```python
from build123d import *

# Parameters (mm, degrees)
F0_R     = 1.6
F1_DEPTH = 3.175


with BuildPart() as f1:
    # F0 (on Top) → F1 (new body)
    with BuildSketch(Plane.XY):
        with BuildLine():
            ThreePointArc((0, 10), (2.928932, 2.928932), (10, 0))
            Line((10, 0), (46, 0))
            ThreePointArc((46, 0), (49.535534, 1.464466), (51, 5))
            Line((51, 5), (51, 15))
            ThreePointArc((51, 15), (49.535534, 18.535534), (46, 20))
            Line((46, 20), (10, 20))
            ThreePointArc((10, 20), (2.928932, 17.071068), (0, 10))
        make_face()
        with Locations((16, 5)):
            Circle(F0_R, mode=Mode.SUBTRACT)
        with Locations((26, 5)):
            Circle(F0_R, mode=Mode.SUBTRACT)
        with Locations((36, 5)):
            Circle(F0_R, mode=Mode.SUBTRACT)
        with Locations((46, 5)):
            Circle(F0_R, mode=Mode.SUBTRACT)
        Polygon((5.686873, 11.150841), (5.518811, 11.651718), (6.045746, 11.689937), (6.007527, 12.216873), (6.527413, 12.122848), (6.621438, 12.642733), (7.101608, 12.422372), (7.321969, 12.902541), (7.732252, 12.56969), (8.065104, 12.979972), (8.37972, 12.555544), (8.804147, 12.87016), (9.003328, 12.380825), (9.492663, 12.580005), (9.563894, 12.056509), (10.08739, 12.12774), (10.026194, 11.602976), (10.550958, 11.54178), (10.361181, 11.048721), (10.85424, 10.858945), (10.547807, 10.428572), (10.97818, 10.122139), (10.574344, 9.781494), (10.914989, 9.377658), (10.439126, 9.148145), (10.668639, 8.672282), (10.150649, 8.568322), (10.254609, 8.050331), (9.727038, 8.078456), (9.698914, 7.550885), (9.194912, 7.709328), (9.036469, 7.205326), (8.587704, 7.484131), (8.308899, 7.035366), (7.943569, 7.417015), (7.56192, 7.051686), (7.30298, 7.512198), (6.842467, 7.253258), (6.706187, 7.763699), (6.195746, 7.627419), (6.190689, 8.155715), (5.662393, 8.150658), (5.788877, 8.663614), (5.275921, 8.790097), (5.525998, 9.255483), (5.060612, 9.505559), (5.418569, 9.894132), (5.029996, 10.252089), (5.473341, 10.539434), (5.185996, 10.982779), align=None, mode=Mode.SUBTRACT)
        with Locations((16, 15)):
            Circle(F0_R, mode=Mode.SUBTRACT)
        with Locations((26, 15)):
            Circle(F0_R, mode=Mode.SUBTRACT)
        with Locations((36, 15)):
            Circle(F0_R, mode=Mode.SUBTRACT)
        with Locations((46, 15)):
            Circle(F0_R, mode=Mode.SUBTRACT)
    extrude(amount=F1_DEPTH)


solid = f1.part
```
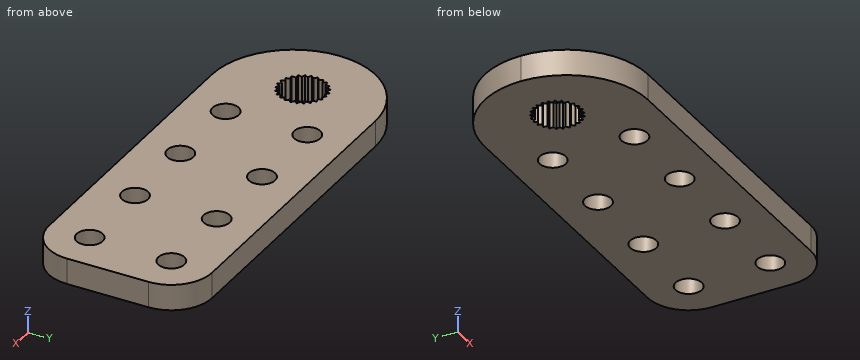
Design review of the part built by this model. Coordinates are the model's own, in mm. Give positions to 0.01 mm unless a question says otherwise; leave off trailing zeros. Write each loop counter-clockwise with the first axis right and the second up, starting at its lowest first coordinate (ties: lowest second). Pieces come first, ordered by that corner, then holes. Notation, with made-up numbers: (-7, 74) - (41, 74) arc R7 cw to (41, 87) - close; hole circle Ø11 at (36.5, -7.5). An arc over 180 degrees is marked (long way). Return JSON: item names as keys, results as strings. Group by question number.
(1) We need section C-C, the plane z = 2.1. Give the number of separate pieces and of enclosed holes in the cut face, then the cut area to 3 significant figures.
(2) To check wall thickness, follow probe 1 along Y at (x, z) = (16, 2.2); probe 2 along Y at (x, z) = (25.5, 0.6); probe 3 along X at (y, z) = (6, 1.2). State the ranges of each line that lie inside material, in increasing order.
(3) We need section B-B, the plane y = 14.25. Give the boundary of the cut face in (x, z) (3 decimals), then the cut area to 3 significant figures.
(4) Insertion check: pin 1 (5 mm diameter, centred on x = 13.5, y = 11.5, fed in from -Z); pin 2 (3 mm diameter, centred on x = 46, y = 15, fed in from +Z); pin 3 (1.5 mm diameter, centred on y = 8.5, z = 1, fed in from -X). Each pin has a flat end and moves straight along its axis. Give the tip position at first contact, or say it passes through.
(5) We need section A-A, the plane x = 26. Give the boundary of the cut face in (y, z) (3 decimals).
Reported:
{
 "1": {"separate pieces": "1", "enclosed holes": "9", "area": "878 mm2"},
 "2": {"probe 1": "y = 0 to 3.4, 6.6 to 13.4, 16.6 to 20", "probe 2": "y = 0 to 3.48, 6.52 to 13.48, 16.52 to 20", "probe 3": "x = 0.83 to 14.75, 17.25 to 24.75, 27.25 to 34.75, 37.25 to 44.75, 47.25 to 51"},
 "3": {"outline": "(0.948, 0) - (14.587, 0) - (14.587, 3.175) - (0.948, 3.175) - close; (17.413, 0) - (24.587, 0) - (24.587, 3.175) - (17.413, 3.175) - close; (27.413, 0) - (34.587, 0) - (34.587, 3.175) - (27.413, 3.175) - close; (37.413, 0) - (44.587, 0) - (44.587, 3.175) - (37.413, 3.175) - close; (47.413, 0) - (51, 0) - (51, 3.175) - (47.413, 3.175) - close", "area": "123 mm2"},
 "4": {"pin 1": "stops at z = 0", "pin 2": "passes through", "pin 3": "stops at x = 0.03"},
 "5": {"outline": "(0, 0) - (3.4, 0) - (3.4, 3.175) - (0, 3.175) - close; (6.6, 0) - (13.4, 0) - (13.4, 3.175) - (6.6, 3.175) - close; (16.6, 0) - (20, 0) - (20, 3.175) - (16.6, 3.175) - close"}
}
